from build123d import *

# Parameters (mm, degrees)
GRUNDPLATTE_DEPTH      = 6
SKIZZE2_W              = 15
SKIZZE2_H              = 12
SKIZZE2_H_2            = 6
ZAPFENDURCHBRUCH_DEPTH = 152.940777937
VERRUNDUNG2_R          = 3
VERRUNDUNG3_R          = 6


with BuildPart() as part:
    # Skizze1 → Grundplatte (new body)
    with BuildSketch(Plane(origin=(0, 0, 0), x_dir=(0, 0, -1), z_dir=(1, 0, 0))):
        Polygon((17.5, 5), (-17.5, 5), (-20.386751346, 0), (-45, 0), (-45, 20), (-17.5, 145), (17.5, 145), (45, 20), (45, 0), (20.386751346, 0), align=None)
    extrude(amount=GRUNDPLATTE_DEPTH)

    # Skizze2 → Zapfendurchbruch (cut, through all)
    with BuildSketch(Plane(origin=(6, 0, 0), x_dir=(0, 0, -1), z_dir=(1, 0, 0))):
        with Locations((0, 130)):
            Rectangle(SKIZZE2_W, SKIZZE2_H)
        with Locations((0, 53)):
            Rectangle(SKIZZE2_W, SKIZZE2_H_2)
        with Locations((0, 13)):
            Rectangle(SKIZZE2_W, SKIZZE2_H_2)
    extrude(amount=-ZAPFENDURCHBRUCH_DEPTH, mode=Mode.SUBTRACT)

    # Verrundung2
    verrundung2_edges = [part.edges().sort_by_distance(p)[0] for p in [
        (3, 0, 20.386751346),
        (3, 0, 45),
        (3, 0, -45),
        (3, 0, -20.386751346),
    ]]
    fillet(verrundung2_edges, radius=VERRUNDUNG2_R)

    # Verrundung3
    verrundung3_edges = [part.edges().sort_by_distance(p)[0] for p in [
        (3, 20, 45),
        (3, 145, 17.5),
        (3, 145, -17.5),
        (3, 20, -45),
    ]]
    fillet(verrundung3_edges, radius=VERRUNDUNG3_R)


solid = part.part
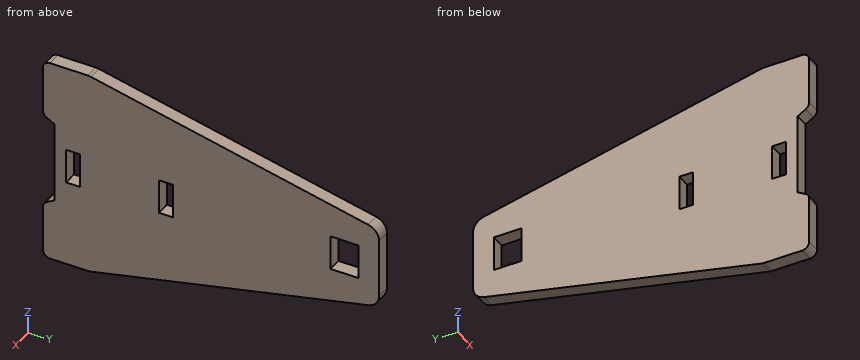
Design review of the part built by this model. Coordinates are the model's own, in mm. Round coordinates to 2 decimals unless told otherwise and drop trailing zeros. Loops run counter-clockwise (first coordinate to the right, second up) from the corner with the lowest first, then second, coordinate; pieces in that order, holes last. Notation, with made-up numbers: (46.5, 34) -> (89.5, 34) arc R25 ccw to (89.5, 58) -> close; hole circle Ø9 at (26.5, 9.25). An arc over 180 degrees is marked (long way). Use one line per item in the form item = value. Start each with the question number.
Q1. We need section C-C on x = 2.8. State how many separate pieces and enclosed holes the cut face has, then the cut area to 3 significant figures.
Q2. We need section A-A on y = 53. Give the boundary of the cut face in (x, z), then the cut area to 3 significant figures.
Q3. For pin 1 Ø2 at (x, y) = (3, 113) entering from +Z; pin 2 Ø1.8 at (x, z) = (2.5, 3) entering from -Y; pin 3 Ø3 at (x, y) = (2.5, 54) entering from +Z, all flat-tipped, find the tip position at first contact; note any pin that passes through.
Q4. We need section D-D on y = 127.5. Give the boundary of the cut face in (x, z).
Q5. We need section B-B on z = 2. Give the boundary of the cut face in (x, y), then the cut area to 3 significant figures.
Q6. Wall thickness on line 1 along Y through (x, z) = (5.3, 5); line 2 along Z through (x, y) = (1.2, 11.5); line 3 along Z through (x, y) = (2.4, 20.5): over which ranges is each line inside the solid? List them lowest first. Write a range as [from, to].
Calculated:
q1.separate_pieces = 1
q1.enclosed_holes = 3
q1.area = 9,050 mm²
q2.outline = (0, -37.74) -> (6, -37.74) -> (6, -7.5) -> (0, -7.5) -> close; (0, 7.5) -> (6, 7.5) -> (6, 37.74) -> (0, 37.74) -> close
q2.area = 363 mm²
q3.pin_1 = 24.76
q3.pin_2 = 5
q3.pin_3 = 37.85
q4.outline = (0, -21.35) -> (6, -21.35) -> (6, -7.5) -> (0, -7.5) -> close; (0, 7.5) -> (6, 7.5) -> (6, 21.35) -> (0, 21.35) -> close
q5.outline = (0, 5) -> (6, 5) -> (6, 10) -> (0, 10) -> close; (0, 16) -> (6, 16) -> (6, 50) -> (0, 50) -> close; (0, 56) -> (6, 56) -> (6, 124) -> (0, 124) -> close; (0, 136) -> (6, 136) -> (6, 145) -> (0, 145) -> close
q5.area = 696 mm²
q6.line_1 = [5, 10], [16, 50], [56, 124], [136, 145]
q6.line_2 = [-45, -7.5], [7.5, 45]
q6.line_3 = [-44.89, 44.89]
